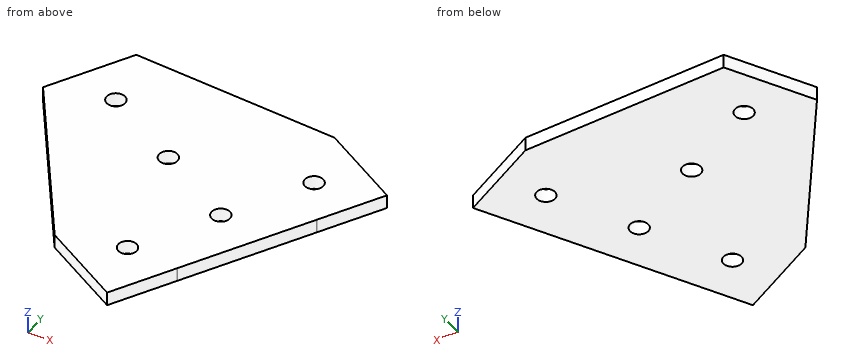
from build123d import *

# Parameters (mm, degrees)
SKETCH_1_R      = 2
EXTRUDE_1_DEPTH = 3


with BuildPart() as part:
    # 草图1 → 凸台-拉伸1 (new body)
    with BuildSketch(Plane.XY):
        with BuildLine():
            Line((14.263569054, -6.979512092), (29.170512591, 18.8400715))
            ThreePointArc((29.170512591, 18.8400715), (29.193213203, 18.880689143), (29.216290822, 18.921093774))
            Line((29.216290822, 18.921093774), (36.716290822, 31.91147483))
            Line((36.716290822, 31.91147483), (19.395782747, 41.91147483))
            Line((19.395782747, 41.91147483), (-25.245233405, 44.590966755))
            Line((-25.245233405, 44.590966755), (-35.245233405, 27.270458679))
            Line((-35.245233405, 27.270458679), (-10.604217253, -10.050049397))
            Line((-10.604217253, -10.050049397), (6.716290822, -20.050049397))
            Line((6.716290822, -20.050049397), (14.216290822, -7.05966834))
            ThreePointArc((14.216290822, -7.05966834), (14.23974345, -7.01948022), (14.263569054, -6.979512092))
        make_face()
        with Locations((-21.584979367, 30.930712717)):
            Circle(SKETCH_1_R, mode=Mode.SUBTRACT)
        with Locations((3.056036785, -6.389795359)):
            Circle(SKETCH_1_R, mode=Mode.SUBTRACT)
        with Locations((13.056036785, 10.930712717)):
            Circle(SKETCH_1_R, mode=Mode.SUBTRACT)
        with Locations((23.056036785, 28.251220792)):
            Circle(SKETCH_1_R, mode=Mode.SUBTRACT)
        with Locations((-4.264471291, 20.930712717)):
            Circle(SKETCH_1_R, mode=Mode.SUBTRACT)
    extrude(amount=EXTRUDE_1_DEPTH)


solid = part.part
Part model, mm, in its own coordinate system. Give positions to 0.01 mm unless a question says otherwise; leave off trailing zeros. Loops run counter-clockwise (first coordinate to the right, second up) from the corner with the lowest first, then second, coordinate; pieces in that order, holes last.
(1) Band-saw the part on C-C (x = 3). Write the cut outline in (y, z), and give its area (3 significant figures).
Return value:
outline: (-17.9, 0) - (-8.39, 0) - (-8.39, 3) - (-17.9, 3) - close; (-4.39, 0) - (42.9, 0) - (42.9, 3) - (-4.39, 3) - close
area: 170 mm2
(2) Drill centre lines: line 1 along X through (y, z) = (29.5, 0.4); line 2 along X through (y, z) = (27, 2.35); line 3 along Y through (x, z) = (24.5, 1.5). Where is each one in solid material? Low to high.
Return value:
line 1: x = -33.96 to -22.98, -20.19 to 21.49, 24.62 to 35.32
line 2: x = -35.07 to 21.5, 24.62 to 33.88
line 3: y = 10.75 to 26.87, 29.64 to 38.96
(3) Band-saw the part on A-A (x = 22.5). Write the cut outline in (y, z).
Return value:
outline: (7.29, 0) - (26.33, 0) - (26.33, 3) - (7.29, 3) - close; (30.17, 0) - (40.12, 0) - (40.12, 3) - (30.17, 3) - close
(4) Band-saw the part on D-D (y = 8). Write the cut outline in (x, z), and give its area (3 significant figures).
Return value:
outline: (-22.52, 0) - (22.91, 0) - (22.91, 3) - (-22.52, 3) - close
area: 136 mm2
(5) Pin check, flat tip, straight feed: pin 1 (1 mm diameter, centred on y = 26, z = 1.5, fed in from -X). Stop position of the tip, or through.
Return value:
pin 1: stops at x = -34.74
(6) Band-saw the part on B-B (z = 1.65). Write the cut outline in (x, y), and give its area (3 significant figures).
Return value:
outline: (-35.25, 27.27) - (-10.6, -10.05) - (6.72, -20.05) - (14.22, -7.06) arc R5 cw to (14.26, -6.98) - (29.17, 18.84) arc R5 cw to (29.22, 18.92) - (36.72, 31.91) - (19.4, 41.91) - (-25.25, 44.59) - close; hole circle Ø4 at (-21.58, 30.93); hole circle Ø4 at (-4.26, 20.93); hole circle Ø4 at (3.06, -6.39); hole circle Ø4 at (13.06, 10.93); hole circle Ø4 at (23.06, 28.25)
area: 2,740 mm2
